Geometry: final body of the model. Coordinates: model frame, mm. Face numbers are marked on the shaded views. A direction names the side the tool comes from. Coordinates: 2 decimals unless noted, no trailing zeros. Order: outer loops, then holes, each group sorted by start corner. A loop starts at its lowest first (then second) coordinate and runs counter-clockwise, first axis right, second up. Notation, with made-up numbers: (76, 88) - (93, 88) arc R11 cw to (93, 94) - close; hole circle Ø6 at (70.25, 57). An arc over 180 degrees is marked (long way). Use a Markdown table: item, result. Add a question column.
Autodesk Inventor part; units mm, degrees
ref_plane "YZ Plane" through (0, 0, 0) normal (1, 0, 0) x (0, 1, 0)
ref_plane "XZ Plane" through (0, 0, 0) normal (0, 1, 0) x (-1, 0, 0)
ref_plane "XY Plane" through (0, 0, 0) normal (0, 0, 1) x (1, 0, 0)
sketch "Sketch1" plane through (0, 0, 0) normal (0, 0, 1) x (1, 0, 0)
  line L0 (-23.4921, 12.3401) -> (-21.4921, 12.3401)
  line L1 (-21.4921, 12.3401) -> (-21.4921, -27.6599)
  line L2 (-21.4921, -27.6599) -> (-23.4921, -27.6599)
  line L3 (-23.4921, -27.6599) -> (-23.4921, 12.3401)
  line L4 (-23.4921, -27.6599) -> (-17.4921, -27.6599)
  line L5 (-17.4921, -27.6599) -> (-17.4921, -25.6599)
  line L6 (-17.4921, -25.6599) -> (-23.4921, -25.6599)
  line L7 (-23.4921, -25.6599) -> (-23.4921, -27.6599)
  line L8 (-17.4921, -27.6599) -> (-19.4921, -27.6599)
  line L9 (-19.4921, -27.6599) -> (-19.4921, -22.6599)
  line L10 (-19.4921, -22.6599) -> (-17.4921, -22.6599)
  line L11 (-17.4921, -22.6599) -> (-17.4921, -27.6599)
  line L12 (-23.4921, 12.3401) -> (-17.4921, 12.3401)
  line L13 (-17.4921, 12.3401) -> (-17.4921, 10.3401)
  line L14 (-17.4921, 10.3401) -> (-23.4921, 10.3401)
  line L15 (-23.4921, 10.3401) -> (-23.4921, 12.3401)
  line L16 (-17.4921, 12.3401) -> (-19.4921, 12.3401)
  line L17 (-19.4921, 12.3401) -> (-19.4921, 7.3401)
  line L18 (-19.4921, 7.3401) -> (-17.4921, 7.3401)
  line L19 (-17.4921, 7.3401) -> (-17.4921, 12.3401)
  line L20 (-19.4921, 9.3401) -> (17.5079, 9.3401)
  line L21 (17.5079, 9.3401) -> (17.5079, 7.3401)
  line L22 (17.5079, 7.3401) -> (-19.4921, 7.3401)
  line L23 (-19.4921, 7.3401) -> (-19.4921, 9.3401)
  line L24 (17.5079, 7.3401) -> (15.5079, 7.3401)
  line L25 (15.5079, 7.3401) -> (15.5079, 12.3401)
  line L26 (15.5079, 12.3401) -> (17.5079, 12.3401)
  line L27 (17.5079, 12.3401) -> (17.5079, 7.3401)
  line L28 (15.5079, 12.3401) -> (21.5079, 12.3401)
  line L29 (21.5079, 12.3401) -> (21.5079, 10.3401)
  line L30 (21.5079, 10.3401) -> (15.5079, 10.3401)
  line L31 (15.5079, 10.3401) -> (15.5079, 12.3401)
  line L32 (21.5079, 12.3401) -> (19.5079, 12.3401)
  line L33 (19.5079, 12.3401) -> (19.5079, -27.6599)
  line L34 (19.5079, -27.6599) -> (21.5079, -27.6599)
  line L35 (21.5079, -27.6599) -> (21.5079, 12.3401)
  line L36 (21.5079, -27.6599) -> (15.5079, -27.6599)
  line L37 (15.5079, -27.6599) -> (15.5079, -25.7551)
  line L38 (15.5079, -25.7551) -> (21.5079, -25.7551)
  line L39 (21.5079, -25.7551) -> (21.5079, -27.6599)
  line L40 (15.5079, -27.6599) -> (17.5079, -27.6599)
  line L41 (17.5079, -27.6599) -> (17.5079, -21.4921)
  line L42 (17.5079, -21.4921) -> (15.5079, -21.4921)
  line L43 (15.5079, -21.4921) -> (15.5079, -27.6599)
  point P0 (0, 0)
  dimension "d0" = 40
  dimension "d1" = 2
  dimension "d2" = 2
  dimension "d3" = 2
  dimension "d4" = 2
  dimension "d5" = 5
  dimension "d6" = 5
  dimension "d7" = 37
  dimension "d8" = 6
  dimension "d9" = 6
  dimension "d10" = 2
  dimension "d11" = 2
  dimension "d12" = 2
  dimension "d13" = 2
  dimension "d14" = 2
  dimension "d15" = 40
  dimension "d16" = 6
  dimension "d17" = 6
  dimension "d18" = 45
extrude "Extrusion1" add sketch "Sketch1" along normal blind 10
sketch "Sketch2" plane through (-17.4921, 9.3401, 0) normal (1, 0, 0) x (0, 0, -1)
  line L0 (-10, 0) -> (0, 0)
  line L1 (0, 3) -> (-10, 3)
  point P0 (0, -9.3401)
  dimension "d21" = 3
sketch "Sketch3" plane through (-17.4921, 9.3401, 0) normal (0, 1, 0) x (1, 0, 0)
  line L0 (-2, -10) -> (35, -10)
  line L1 (5, 0) -> (8, 0)
  line L2 (8, 0) -> (8, -10)
  line L3 (8, -10) -> (5, -10)
  line L4 (5, -10) -> (5, 0)
  line L5 (28, 0) -> (25, 0)
  line L6 (25, 0) -> (25, -10)
  line L7 (25, -10) -> (28, -10)
  line L8 (28, -10) -> (28, 0)
  line L9 (0, 0) -> (0, -10)
  line L10 (33, 0) -> (33, -10)
  point P0 (17.4921, 0)
  dimension "d22" = 5
  dimension "d23" = 5
  dimension "d24" = 3
  dimension "d25" = 3
extrude "Extrusion2" add sketch "Sketch3" along normal blind 3
properties part number "Up go er"
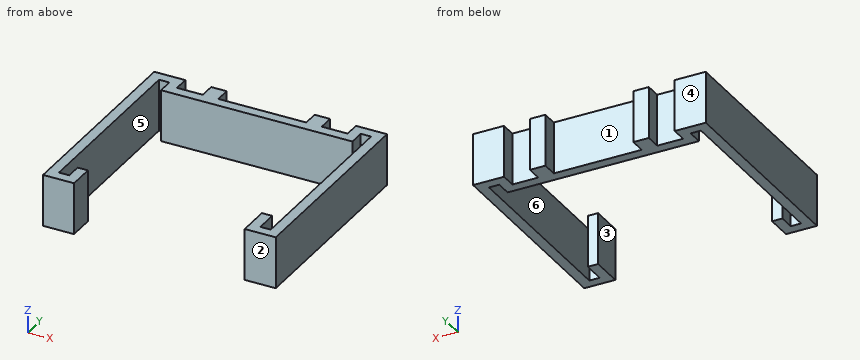
1) Ray query, line 1 along X through (y, z) = (-22, 4.5); line 2 along X through (y, z) = (-9.5, 5.25); line 3 along X through (y, z) = (8, 1.25). Return the intervals inside material, ascending.
2) Set-up query: the marked faces 1 and 2. Return all of +Z, -Z, +X, -X, +Y, -Y with unobstructed straight access to the full face (end or side cutting, diameter ignored); none if empty.
3) Pin query (flat end, axial travel): pin 1 (5 mm diameter, centred on x = 7.5, z = 7.5, fed in from -Y); pin 2 (2 mm diameter, centred on x = -15.5, z = 8.5, fed in from +Y); pin 3 (5 mm diameter, centred on x = 15.5, y = 2, fed in from -Z). Return the tip coordinate at first contact, or that it passes through.
4) Section D-D (x = 15). Return loops of the section in (y, z), then the cut area to 3 significant figures.
5) Draft query along Y for the marked faces 3, 4, 5 and 6. Return one class per face: pulls with the +Y half, pulls with the -Y half, needs draft (parallel to the pull), parting line crosses it, or undercut.
6) Section A-A (y = -2.5). Return loops of the section in (x, z).
7) Section C-C (x = -11). Return loops of the section in (y, z).
Values follow:
| question | item | result |
|---|---|---|
| 1 | line 1 | x = -23.49 to -21.49, 15.51 to 17.51, 19.51 to 21.51 |
| 1 | line 2 | x = -23.49 to -21.49, 19.51 to 21.51 |
| 1 | line 3 | x = -23.49 to -21.49, -19.49 to 17.51, 19.51 to 21.51 |
| 2 | face 1 | +Z, -Z, +Y |
| 2 | face 2 | +Z, -Z, +X, -X, -Y |
| 3 | pin 1 | stops at y = 7.34 |
| 3 | pin 2 | stops at y = 9.34 |
| 3 | pin 3 | passes through |
| 4 | outline | (7.34, 0) - (9.34, 0) - (9.34, 10) - (7.34, 10) - close |
| 4 | area | 20.0 mm² |
| 5 | face 3 | needs draft |
| 5 | face 4 | pulls with the +Y half |
| 5 | face 5 | undercut |
| 5 | face 6 | undercut |
| 6 | outline | (-23.49, 0) - (-21.49, 0) - (-21.49, 10) - (-23.49, 10) - close; (19.51, 0) - (21.51, 0) - (21.51, 10) - (19.51, 10) - close |
| 7 | outline | (7.34, 0) - (12.34, 0) - (12.34, 10) - (7.34, 10) - close |
